Could you check a few things on this model? Use its own coordinates, in mm. Face numbers are marked on the shaded views. A direction names the side the tool comes from. Round coordinates to 2 decimals unless told otherwise and drop trailing zeros. Write each loop counter-clockwise with the first axis right and the second up, starting at its lowest first coordinate (ties: lowest second). Pieces come first, ordered by that corner, then holes. Notation, with made-up numbers: (29.5, 65.5) -> (58.5, 65.5) arc R29 ccw to (58.5, 94.5) -> close; hole circle Ø5 at (13, -18.5). An arc over 180 degrees is marked (long way). Return JSON: item names as keys, results as strings.
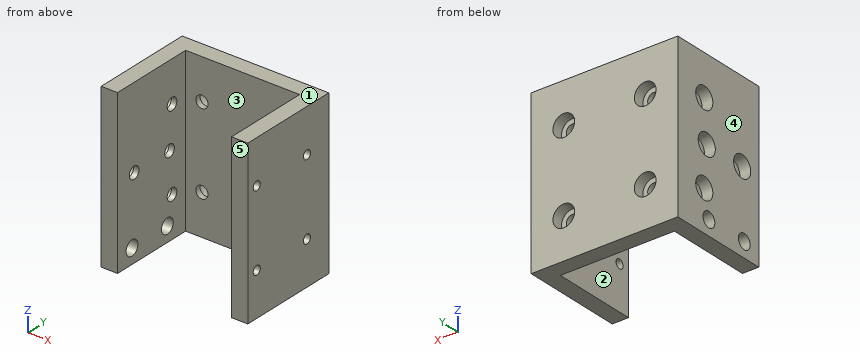
from build123d import *

# Parameters (mm, degrees)
SKETCH1_W                      = 54
SKETCH1_H                      = 37.75
BOSS_EXTRUDE1_DEPTH            = 30
SKETCH2_W                      = 42
SKETCH2_H                      = 31.75
CUT_EXTRUDE1_DEPTH             = 76.855537042
CBORE_FOR_M4_SHCS1_D           = 4.5
CBORE_FOR_M4_SHCS1_DEPTH       = 6
CBORE_FOR_M4_SHCS1_CBORE_D     = 8
CBORE_FOR_M4_SHCS1_CBORE_DEPTH = 4
M5_CLEARANCE_HOLE1_D           = 5.5
M5_CLEARANCE_HOLE1_DEPTH       = 6
CBORE_START                    = 33.75
CBORE_FOR_M4_SHCS2_OUTLINE_R   = 4
CBORE_FOR_M4_SHCS2_DEPTH       = 4
CBORE_START_2                  = 31.75
CBORE_FOR_M4_SHCS2_2_OUTLINE_R = 2.25
CBORE_FOR_M4_SHCS2_2_DEPTH     = 2
M4X0_7_START                   = 21
M4X0_7_TAPPED_HOLE1_OUTLINE_R  = 1.65
M4X0_7_TAPPED_HOLE1_DEPTH      = 6


# Read off the part's stored shape, not the designer's step: CBORE for M4 SHCS2, M4x0.7 Tapped Hole1
with BuildPart() as part:
    # Sketch1 → Boss-Extrude1 (new, symmetric)
    with BuildSketch(Plane.XY):
        with Locations((0, 18.875)):
            Rectangle(SKETCH1_W, SKETCH1_H)
    extrude(amount=BOSS_EXTRUDE1_DEPTH, both=True)

    # Sketch2 → Cut-Extrude1 (cut, through all)
    with BuildSketch(Plane.XY.offset(30)):
        with Locations((0, 15.875)):
            Rectangle(SKETCH2_W, SKETCH2_H)
    extrude(amount=-CUT_EXTRUDE1_DEPTH, mode=Mode.SUBTRACT)

    # CBORE for M4 SHCS1
    with Locations(Plane.ZY.offset(27)):
        with Locations((15, 25.4), (0, 24.25), (0, 7.75), (-15, 25.4)):
            CounterBoreHole(CBORE_FOR_M4_SHCS1_D / 2, CBORE_FOR_M4_SHCS1_CBORE_D / 2, CBORE_FOR_M4_SHCS1_CBORE_DEPTH, depth=CBORE_FOR_M4_SHCS1_DEPTH)

    # M5 Clearance Hole1
    with Locations(Plane.ZY.offset(27)):
        with Locations((-24.5, 23.25), (-24.5, 6.75)):
            Hole(M5_CLEARANCE_HOLE1_D / 2, depth=M5_CLEARANCE_HOLE1_DEPTH)

    # CBORE for M4 SHCS2 outline → CBORE for M4 SHCS2 (cut)
    with BuildSketch(Plane(origin=(0, 0, 0), x_dir=(1, 0, 0), z_dir=(0, 1, 0)).offset(CBORE_START)):
        with Locations((15, 15)):
            Circle(CBORE_FOR_M4_SHCS2_OUTLINE_R)
        with Locations((-15, -15)):
            Circle(CBORE_FOR_M4_SHCS2_OUTLINE_R)
        with Locations((-15, 15)):
            Circle(CBORE_FOR_M4_SHCS2_OUTLINE_R)
        with Locations((15, -15)):
            Circle(CBORE_FOR_M4_SHCS2_OUTLINE_R)
    extrude(amount=CBORE_FOR_M4_SHCS2_DEPTH, mode=Mode.SUBTRACT)

    # CBORE for M4 SHCS2 2 outline → CBORE for M4 SHCS2 2 (cut)
    with BuildSketch(Plane(origin=(0, 0, 0), x_dir=(1, 0, 0), z_dir=(0, 1, 0)).offset(CBORE_START_2)):
        with Locations((15, 15)):
            Circle(CBORE_FOR_M4_SHCS2_2_OUTLINE_R)
        with Locations((-15, -15)):
            Circle(CBORE_FOR_M4_SHCS2_2_OUTLINE_R)
        with Locations((-15, 15)):
            Circle(CBORE_FOR_M4_SHCS2_2_OUTLINE_R)
        with Locations((15, -15)):
            Circle(CBORE_FOR_M4_SHCS2_2_OUTLINE_R)
    extrude(amount=CBORE_FOR_M4_SHCS2_2_DEPTH, mode=Mode.SUBTRACT)

    # M4x0.7 Tapped Hole1 outline → M4x0.7 Tapped Hole1 (cut)
    with BuildSketch(Plane.YZ.offset(M4X0_7_START)):
        with Locations((27.575, 14)):
            Circle(M4X0_7_TAPPED_HOLE1_OUTLINE_R)
        with Locations((4.175, -14)):
            Circle(M4X0_7_TAPPED_HOLE1_OUTLINE_R)
        with Locations((27.575, -14)):
            Circle(M4X0_7_TAPPED_HOLE1_OUTLINE_R)
        with Locations((4.175, 14)):
            Circle(M4X0_7_TAPPED_HOLE1_OUTLINE_R)
    extrude(amount=M4X0_7_TAPPED_HOLE1_DEPTH, mode=Mode.SUBTRACT)


solid = part.part
1) I want a section at D-D, the plane x = 22.5. Please give me the cut outline in (y, z) (3 decimals).
Return value:
{"outline": "(0, -30) -> (37.75, -30) -> (37.75, 30) -> (0, 30) -> close; hole circle Ø3.3 at (4.175, -14); hole circle Ø3.3 at (4.175, 14); hole circle Ø3.3 at (27.575, -14); hole circle Ø3.3 at (27.575, 14)"}
2) I want a section at B-B, the plane y = 30.5. Please give me the cut outline in (x, z), and give its area (3 significant figures).
Return value:
{"outline": "(-27, -30) -> (-21, -30) -> (-21, 30) -> (-27, 30) -> close; (21, -30) -> (27, -30) -> (27, 30) -> (21, 30) -> close", "area": "720 mm²"}
3) Will these pins go through, and if not, where does the flat tip stop? pin 1 Ø9 at (x, z) = (14.5, 15.5) entering from +Y; pin 2 Ø2.5 at (y, z) = (25.4, -15) entering from -X; pin 3 Ø1.5 at (x, y) = (-20, 16) entering from -Z; pin 4 Ø3 at (x, z) = (1, -8.5) entering from -Y.
Return value:
{"pin 1": "y = 37.75", "pin 2": "x = 21", "pin 3": "through", "pin 4": "y = 31.75"}
4) I want a section at A-A, the plane z = 0. Please give me the cut outline in (x, y), and give its area (3 significant figures).
Return value:
{"outline": "(-27, 0) -> (-21, 0) -> (-21, 5.5) -> (-23, 5.5) -> (-23, 3.75) -> (-27, 3.75) -> close; (-27, 11.75) -> (-23, 11.75) -> (-23, 10) -> (-21, 10) -> (-21, 22) -> (-23, 22) -> (-23, 20.25) -> (-27, 20.25) -> close; (-27, 28.25) -> (-23, 28.25) -> (-23, 26.5) -> (-21, 26.5) -> (-21, 31.75) -> (21, 31.75) -> (21, 0) -> (27, 0) -> (27, 37.75) -> (-27, 37.75) -> close", "area": "623 mm²"}
5) For the marked faces 1 and 2, which set-ups out of +Z, -Z, +X, -X, +Y, -Y let a thin tool reach every point of the face, with its end or its side?
Return value:
{"face 1": "+Z, +X, -X, +Y, -Y", "face 2": "+Z, -Z, -Y"}
6) I want a section at C-C, the plane x = 15. Please give me the cut outline in (y, z).
Return value:
{"outline": "(31.75, -30) -> (37.75, -30) -> (37.75, -19) -> (33.75, -19) -> (33.75, -17.25) -> (31.75, -17.25) -> close; (31.75, -12.75) -> (33.75, -12.75) -> (33.75, -11) -> (37.75, -11) -> (37.75, 11) -> (33.75, 11) -> (33.75, 12.75) -> (31.75, 12.75) -> close; (31.75, 17.25) -> (33.75, 17.25) -> (33.75, 19) -> (37.75, 19) -> (37.75, 30) -> (31.75, 30) -> close"}
7) If I drill on probe 1 along X at (y, z) = (32.65, 15); probe 2 along Z at (x, y) = (-15, 32); probe 3 along Y at (x, z) = (-21.95, 0), over which ranges is the centre line in solid material (lowest first)? Write a range as [from, to].
Return value:
{"probe 1": "[-27, -17.25], [-12.75, 12.75], [17.25, 27]", "probe 2": "[-30, -17.25], [-12.75, 12.75], [17.25, 30]", "probe 3": "[0, 5.5], [10, 22], [26.5, 37.75]"}
8) Thinking about a two-plate mould opening in X: for the marked faces 3, 4 and 5, which applies, pulls with the +X half, pulls with the -X half, needs draft (parallel to the pull), parting line crosses it, or undercut?
Return value:
{"face 3": "undercut", "face 4": "pulls with the -X half", "face 5": "needs draft"}
